Could you check a few things on this model? Use its own coordinates, in mm. Face numbers are marked on the shaded views. A direction names the side the tool comes from. Coordinates: 2 decimals unless noted, no trailing zeros. Order: outer loops, then holes, each group sorted by start corner. A loop starts at its lowest first (then second) coordinate and runs counter-clockwise, first axis right, second up. Notation, with made-up numbers: (-18, 68.5) -> (19, 68.5) arc R26 cw to (19, 87.5) -> close; hole circle Ø3 at (-29, 5.25). An arc over 180 degrees is marked (long way). Use a Markdown table: item, result. Add a question column.
1) If we section it at B-B (z = 0): Write out the boundary of the cut face in (x, y).
2) Thinking about a two-plate mould opening in Y: for the marked faces 3, 4, 5 and 6, which applies, +Y half, -Y half, draft (parallel to the pull), parting line (faces both ways), or undercut?
3) If I drill on L1, parallel to Y at x = 0, z = 2.3; L2, parallel to Z at x = 3, y = 0; L3, parallel to X at y = 4, z = -1.35, over which ranges is the centre line in solid material (lowest first)? Write a range as [from, to].
4) If we section it at D-D (x = 1.25): Write out the boundary of the cut face in (y, z).
5) Which directions (+Z, -Z, +X, -X, +Y, -Y) give clear straight access to the entire face, cutting with the end or side of a thin tool? Please do the marked faces 1 and 2.
6) Will these pins go through, and if not, where does the flat tip stop? pin 1 Ø3 at (y, z) = (0, 0) entering from +X; pin 2 Ø3 at (x, z) = (-2.5, 0.5) entering from -Y.
7) If we section it at C-C (x = 0.5): Write out the boundary of the cut face in (y, z).
8) If we section it at A-A (y = 0): Write out the boundary of the cut face in (x, z), plus the area to 3 significant figures.
```python
from build123d import *

# Parameters (mm, degrees)
EXTRUDE_1_DEPTH     = 3
SKETCH_2_R          = 1.65
CUT_EXTRUDE_2_DEPTH = 23
SKETCH_3_R          = 1.1
CUT_EXTRUDE_3_DEPTH = 23
SKETCH_4_R          = 1.1
CUT_EXTRUDE_4_DEPTH = 23


with BuildPart() as part:
    # 草图1 → 凸台-拉伸1 (new, symmetric)
    with BuildSketch(Plane.XY):
        with BuildLine():
            Line((-3.5, -4), (-3.5, 4))
            ThreePointArc((-3.5, 4), (0, 7.5), (3.5, 4))
            Line((3.5, 4), (3.5, -4))
            ThreePointArc((3.5, -4), (0, -7.5), (-3.5, -4))
        make_face()
    extrude(amount=EXTRUDE_1_DEPTH, both=True)

    # 草图2 → 切除-拉伸2 (cut)
    with BuildSketch(Plane(origin=(3.5, 0, 0), x_dir=(0, 0, -1), z_dir=(1, 0, 0))):
        Circle(SKETCH_2_R)
        Polygon((-0.730979877, 1.479245895), (-1.405289173, 9.186636415), (1.405289173, 9.186636415), (0.730979877, 1.479245895), (0, 1.479245895), align=None)
    extrude(amount=-CUT_EXTRUDE_2_DEPTH, mode=Mode.SUBTRACT)

    # 草图3 → 切除-拉伸3 (cut)
    with BuildSketch(Plane.XY.offset(3)):
        with Locations((0, 4)):
            Circle(SKETCH_3_R)
    extrude(amount=-CUT_EXTRUDE_3_DEPTH, mode=Mode.SUBTRACT)

    # 草图4 → 切除-拉伸4 (cut)
    with BuildSketch(Plane.XY.offset(3)):
        with Locations((0, -4)):
            Circle(SKETCH_4_R)
    extrude(amount=-CUT_EXTRUDE_4_DEPTH, mode=Mode.SUBTRACT)


solid = part.part
```
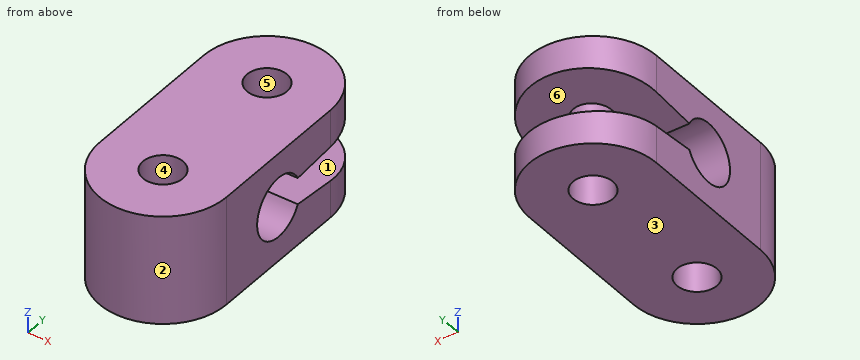
Answer sheet:
| question | item | result |
|---|---|---|
| 1 | outline | (-3.5, -4) arc R3.5 ccw to (3.5, -4) -> (3.5, -1.65) -> (-3.5, -1.65) -> close; hole circle Ø2.2 at (0, -4) |
| 2 | face 3 | draft |
| 2 | face 4 | undercut |
| 2 | face 5 | undercut |
| 2 | face 6 | +Y half |
| 3 | L1 | [-7.5, -5.1], [-2.9, 2.9], [5.1, 7.5] |
| 3 | L2 | [-3, -1.65], [1.65, 3] |
| 3 | L3 | [-3.5, -1.1], [1.1, 3.5] |
| 4 | outline | (-7.27, -3) -> (7.27, -3) -> (7.27, -1.24) -> (1.48, -0.73) arc R1.65 cw (long way) to (1.48, 0.73) -> (7.27, 1.24) -> (7.27, 3) -> (-7.27, 3) -> close |
| 5 | face 1 | +X, -X, +Y |
| 5 | face 2 | +Z, -Z, -Y |
| 6 | pin 1 | through |
| 6 | pin 2 | y = -7.35 |
| 7 | outline | (-7.46, -3) -> (-4.98, -3) -> (-4.98, 3) -> (-7.46, 3) -> close; (-3.02, -3) -> (3.02, -3) -> (3.02, -0.87) -> (1.48, -0.73) arc R1.65 cw (long way) to (1.48, 0.73) -> (3.02, 0.87) -> (3.02, 3) -> (-3.02, 3) -> close; (4.98, -3) -> (7.46, -3) -> (7.46, -1.25) -> (4.98, -1.04) -> close; (4.98, 1.04) -> (7.46, 1.25) -> (7.46, 3) -> (4.98, 3) -> close |
| 8 | outline | (-3.5, -3) -> (3.5, -3) -> (3.5, -1.65) -> (-3.5, -1.65) -> close; (-3.5, 1.65) -> (3.5, 1.65) -> (3.5, 3) -> (-3.5, 3) -> close |
| 8 | area | 18.9 mm2 |
